Source: CAD feature listing. Evaluate the final solid. Frame: model axes, mm. Face numbers are marked on the shaded views. A direction names the side the tool comes from. Coordinates: 2 decimals unless noted, no trailing zeros. Loops run counter-clockwise (first coordinate to the right, second up) from the corner with the lowest first, then second, coordinate; pieces in that order, holes last.
Item 1: Section query A-A, the plane z = -42.75. Return the cut outline in (x, y).
Item 2: Pull-direction query (Y, two-part tool) for the marked faces 1, 2 and 3; classes: +Y half, -Y half, draft (parallel to the pull), parting line (faces both ways), or undercut.
Item 3: Reachability of the marked faces 4 and 5 from +Z, -Z, +X, -X, +Y, -Y: full face, straight path, thin tool, end or side. Return the list, or none.
Item 4: Section query C-C, the plane y = 126. Return the cut outline in (x, z), then the cut area to 3 significant figures.
Item 5: Section query B-B, the plane x = 96. Return the cut outline in (y, z), then the cut area to 3 significant figures.
Item 6: Pin query (flat end, axial travel): pin 1 Ø4 at (x, y) = (164.5, 97.5) entering from +Z; pin 2 Ø1 at (x, z) = (151, -46.5) entering from -Y; pin 3 Ø0.8 at (y, z) = (0.5, -55.5) entering from -X. Return the tip coordinate at first contact, or that it passes through.
Item 7: Line query: probe 1 along Y at (x, z) = (86, -52.25); probe 2 along Z at (x, y) = (154, 145); probe 3 along Y at (x, z) = (191, -55). Output: solid intervals per line, ascending.
Item 8: Section query D-D, the plane x = 46. Return the cut outline in (y, z).
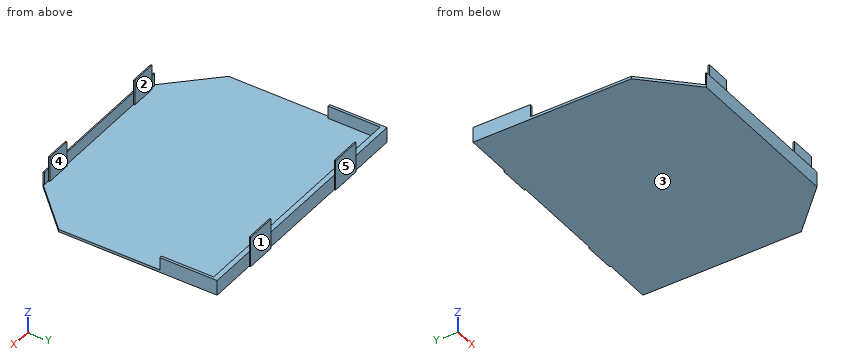
```python
from build123d import *

# Parameters (mm, degrees)
STOCK_PART1_1_START       = -61
STOCK_PART1_1_DEPTH       = 2
STOCK_PART1_1_START_2     = -59
STOCK_PART1_1_2_OUTLINE_W = 130
STOCK_PART1_1_2_OUTLINE_H = 1
STOCK_PART1_1_2_DEPTH     = 10
SKETCH1_W                 = 24
SKETCH1_H                 = 24
BOSS_EXTRUDE1_DEPTH       = 1
SKETCH2_W                 = 20
SKETCH2_H                 = 20
BOSS_EXTRUDE2_DEPTH       = 1


# Read off the part's stored shape, not the designer's step: Stock-Part1-1
with BuildPart() as part:
    # Stock-Part1-1 outline → Stock-Part1-1 (new body)
    with BuildSketch(Plane.XY.offset(STOCK_PART1_1_START)):
        Polygon((0, 35.707142143), (35, 0), (165, 0), (200, 35.707142143), (200, 160), (0, 160), align=None)
    extrude(amount=STOCK_PART1_1_DEPTH)

    # Stock-Part1-1 2 outline → Stock-Part1-1 2 (add)
    with BuildSketch(Plane.XY.offset(STOCK_PART1_1_START_2)):
        with Locations((100, 0.5)):
            Rectangle(STOCK_PART1_1_2_OUTLINE_W, STOCK_PART1_1_2_OUTLINE_H)
        Polygon((198, 115), (200, 115), (200, 160), (0, 160), (0, 115), (2, 115), (2, 156), (198, 156), align=None)
    extrude(amount=STOCK_PART1_1_2_DEPTH)

    # Sketch1 → Boss-Extrude1 (add)
    with BuildSketch(Plane(origin=(0, 160, 0), x_dir=(1, 0, 0), z_dir=(0, 1, 0))):
        with Locations((150, 49)):
            Rectangle(SKETCH1_W, SKETCH1_H)
        with Locations((50, 49)):
            Rectangle(SKETCH1_W, SKETCH1_H)
    extrude(amount=BOSS_EXTRUDE1_DEPTH)

    # Sketch2 → Boss-Extrude2 (add)
    with BuildSketch(Plane(origin=(0, 1, 0), x_dir=(1, 0, 0), z_dir=(0, 1, 0))):
        with Locations((50, 49)):
            Rectangle(SKETCH2_W, SKETCH2_H)
        with Locations((150, 49)):
            Rectangle(SKETCH2_W, SKETCH2_H)
    extrude(amount=BOSS_EXTRUDE2_DEPTH)


solid = part.part
```
Verdict:
1. outline: (38, 160) - (62, 160) - (62, 161) - (38, 161) - close; (40, 1) - (60, 1) - (60, 2) - (40, 2) - close; (138, 160) - (162, 160) - (162, 161) - (138, 161) - close; (140, 1) - (160, 1) - (160, 2) - (140, 2) - close
2. face 1: +Y half
2. face 2: undercut
2. face 3: draft
3. face 4: +Z, +X, -X
3. face 5: +Z, -Z, +X, -X, +Y
4. outline: (0, -61) - (200, -61) - (200, -49) - (198, -49) - (198, -59) - (2, -59) - (2, -49) - (0, -49) - close
4. area: 440 mm2
5. outline: (0, -61) - (160, -61) - (160, -49) - (156, -49) - (156, -59) - (1, -59) - (1, -49) - (0, -49) - close
5. area: 370 mm2
6. pin 1: stops at z = -59
6. pin 2: stops at y = 1
6. pin 3: stops at x = 35
7. probe 1: y = 0 to 1, 156 to 160
7. probe 2: z = -61 to -59
7. probe 3: y = 156 to 160
8. outline: (0, -61) - (161, -61) - (161, -37) - (160, -37) - (160, -49) - (156, -49) - (156, -59) - (2, -59) - (2, -39) - (1, -39) - (1, -49) - (0, -49) - close
